Input: part model. Units: mm. Frame: model coordinates. Coordinates: 2 decimals unless noted, no trailing zeros. Write each loop counter-clockwise with the first axis right and the second up, starting at its lowest first coordinate (ties: lowest second). Pieces come first, ordered by that corner, then holes. Notation, with made-up numbers: M 22,20.25 L 73,20.25 A17 cw 73,53.25 Z; hole C 1.25,-18 d1. An arc over 180 degrees is marked long. Use one line per item in the form item = value.
from build123d import *

# Parameters (mm, degrees)
F1_DEPTH = 25
F2_DEPTH = 10


with BuildPart() as f1:
    # F0 (on Top) → F1 (new body)
    with BuildSketch(Plane.XY):
        Polygon((19.75, 198), (27.75, 198), (35.75, 198), (27.75, 223.787594), align=None)
        Polygon((35.75, 198), (27.75, 198), (19.75, 198), (0, 0), (55.5, 0), align=None)
    extrude(amount=F1_DEPTH)

    # F0 (on Top) → F2 (join)
    with BuildSketch(Plane.XY):
        Polygon((19.75, 198), (27.75, 198), (35.75, 198), (27.75, 223.787594), align=None)
        Polygon((35.75, 198), (27.75, 198), (19.75, 198), (0, 0), (55.5, 0), align=None)
    extrude(amount=F2_DEPTH)


solid = f1.part
(1) Section query C-C on x = 7. Return the cut outline in (y, z), plus the area to 3 significant figures.
Computed:
outline = M 0,0 L 70.18,0 L 70.18,25 L 0,25 Z
area = 1,750 mm^2
(2) Section query B-B on y = 32. Return the cut outline in (x, z).
Computed:
outline = M 3.19,0 L 52.31,0 L 52.31,25 L 3.19,25 Z
(3) Line query: probe 1 along X at (y, z) = (194, 11); probe 2 along X at (y, z) = (53, 10.5). Output: solid intervals per line, ascending.
Computed:
probe_1 = 19.35 to 36.15
probe_2 = 5.29 to 50.21
(4) First-contact query: pin 1 Ø12 at (y, z) = (180.5, 20) entering from -X; pin 2 Ø6 at (y, z) = (107, 15.5) entering from -X; pin 3 Ø2 at (y, z) = (177, 15.5) entering from -X. Flat tips, straight axial feed; report the tip coordinate or a pass-through.
Computed:
pin_1 = 17.41
pin_2 = 10.37
pin_3 = 17.56
(5) Section query A-A on z = 16.5. Return the cut outline in (x, y).
Computed:
outline = M 0,0 L 55.5,0 L 35.75,198 L 27.75,223.79 L 19.75,198 Z
